Print and shaded views of the part. All mm, measured from the part's lowest x, y and z. A direction names the side the tool comes from. Coordinates: 2 decimals unless noted, no trailing zeros. Loops run counter-clockwise (first coordinate to the right, second up) from the corner with the lowest first, then second, coordinate; pieces in that order, holes last. Notation, with made-up numbers: M -23,1.5 L 29,1.5 A18 cw 29,32.5 Z; hole C -9,29.5 d11. An arc over 180 degrees is marked long. Use a Markdown table: item, result. Add a question column.
1) Tool access for the marked faces 1 and 2: list every direction of +Z, -Z, +X, -X, +Y, -Y with a clear straight run to the whole face (end or side of a thin tool).
2) Pin check, flat tips, straight feed: pin 1 Ø2.5 at (x, y) = (5, 5) entering from -Z; pin 2 Ø6 at (x, z) = (4, 24.5) entering from -Y; pin 3 Ø4 at (y, z) = (5.5, 11.5) entering from +X; pin 4 Ø4 at (y, z) = (8, 29.5) entering from +X. Stop position of each tip, or through.
3) Band-saw the part on A-A (y = 5.08). List the corners of the cut face in (x, z), plus the area to 3 significant figures.
4) Band-saw the part on D-D (z = 16). List the corners of the cut face in (x, y), plus the area to 3 significant figures.
5) Band-saw the part on C-C (z = 2). List the corners of the cut face in (x, y).
6) Wall check: probe 1 along Y at (x, z) = (5.08, 6); probe 2 along Z at (x, y) = (2.75, 8.25); probe 3 along Z at (x, y) = (4.75, 2.25). Give the ranges that are in metal, low to high. Write a range as from..to.
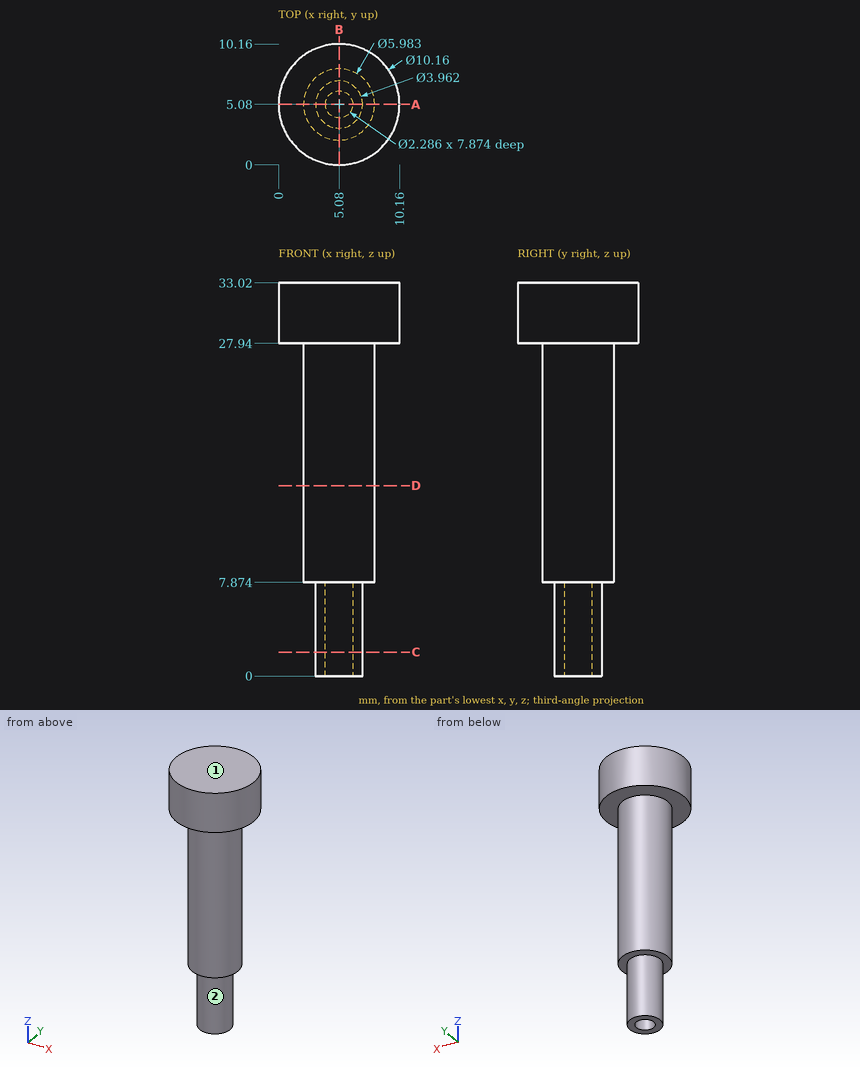
Entries:
| question | item | result |
|---|---|---|
| 1 | face 1 | +Z, +X, -X, +Y, -Y |
| 1 | face 2 | -Z |
| 2 | pin 1 | z = 0 |
| 2 | pin 2 | y = 2.09 |
| 2 | pin 3 | x = 8.07 |
| 2 | pin 4 | x = 10.08 |
| 3 | outline | M 0,27.94 L 2.09,27.94 L 2.09,7.87 L 3.1,7.87 L 3.1,0 L 3.94,0 L 3.94,7.87 L 6.22,7.87 L 6.22,0 L 7.06,0 L 7.06,7.87 L 8.07,7.87 L 8.07,27.94 L 10.16,27.94 L 10.16,33.02 L 0,33.02 Z |
| 3 | area | 185 mm2 |
| 4 | outline | C 5.08,5.08 d5.98 |
| 4 | area | 28.1 mm2 |
| 5 | outline | C 5.08,5.08 d3.96; hole C 5.08,5.08 d2.29 |
| 6 | probe 1 | 3.1..3.94, 6.22..7.06 |
| 6 | probe 2 | 27.94..33.02 |
| 6 | probe 3 | 7.87..33.02 |
